Input: part model. Units: mm. Frame: model coordinates. Face numbers are marked on the shaded views. A direction names the side the tool comes from. Give positions to 0.01 mm unless a question says otherwise; leave off trailing zeros. Loops run counter-clockwise (first coordinate to the right, second up) from the corner with the lowest first, then second, coordinate; pieces in that order, holes last. Notation, with made-up numbers: (44, 10.25) -> (78, 10.25) arc R25 ccw to (78, 48.25) -> close; hole circle Ø11 at (4, 49). An arc over 180 degrees is marked (long way). One line per question, with ' | ' between items.
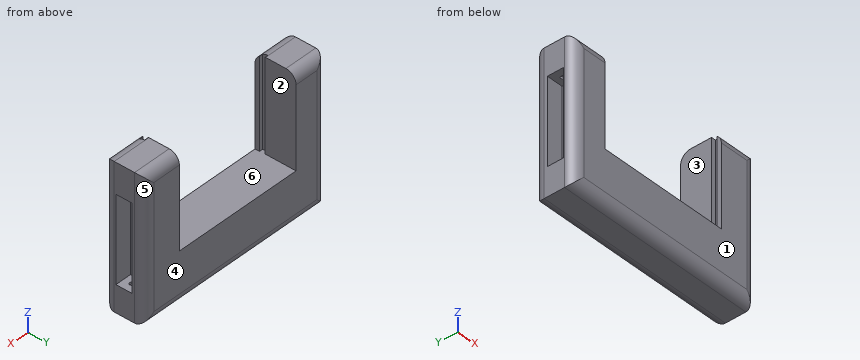
from build123d import *

# Parameters (mm, degrees)
SKETCH1_W           = 50
SKETCH1_H           = 35
BOSS_EXTRUDE1_DEPTH = 10
SKETCH2_W           = 34
SKETCH2_H           = 1.3
CUT_EXTRUDE1_DEPTH  = 22.5
SKETCH3_W           = 15
SKETCH3_H           = 7.598280995
CUT_EXTRUDE2_DEPTH  = 22.5
SKETCH4_W           = 17.2
SKETCH4_H           = 7.598280995
CUT_EXTRUDE3_DEPTH  = 22.5
SKETCH5_W           = 13.5
SKETCH5_H           = 1.101719005
CUT_EXTRUDE4_DEPTH  = 22.5
SKETCH6_W           = 18.6
SKETCH6_H           = 1.101719005
CUT_EXTRUDE5_DEPTH  = 22.5
SKETCH7_W           = 21
SKETCH7_H           = 4
CUT_EXTRUDE6_DEPTH  = 4
SKETCH8_R           = 0.5
CUT_EXTRUDE7_DEPTH  = 0.5
SKETCH9_R           = 0.5
CUT_EXTRUDE8_DEPTH  = 0.5
SKETCH10_W          = 21
SKETCH10_H          = 4
CUT_EXTRUDE9_DEPTH  = 4
SKETCH11_R          = 0.5
CUT_EXTRUDE10_DEPTH = 0.5
SKETCH12_R          = 0.5
CUT_EXTRUDE11_DEPTH = 0.5
FILLET1_R           = 2.5


with BuildPart() as part:
    # Sketch1 → Boss-Extrude1 (new body)
    with BuildSketch(Plane(origin=(0, 0, 0), x_dir=(1, 0, 0), z_dir=(0, 1, 0))):
        with Locations((-1.379996057, -3.323754789)):
            Rectangle(SKETCH1_W, SKETCH1_H)
    extrude(amount=BOSS_EXTRUDE1_DEPTH)

    # Sketch2 → Cut-Extrude1 (cut)
    with BuildSketch(Plane.XY.offset(20.823754789)):
        with Locations((-1.867795916, 1.751719005)):
            Rectangle(SKETCH2_W, SKETCH2_H)
    extrude(amount=-CUT_EXTRUDE1_DEPTH, mode=Mode.SUBTRACT)

    # Sketch3 → Cut-Extrude2 (cut)
    with BuildSketch(Plane.XY.offset(20.823754789)):
        with Locations((6.564825068, 6.200859503)):
            Rectangle(SKETCH3_W, SKETCH3_H)
    extrude(amount=-CUT_EXTRUDE2_DEPTH, mode=Mode.SUBTRACT)

    # Sketch4 → Cut-Extrude3 (cut)
    with BuildSketch(Plane.XY.offset(20.823754789)):
        with Locations((-9.535174932, 6.200859503)):
            Rectangle(SKETCH4_W, SKETCH4_H)
    extrude(amount=-CUT_EXTRUDE3_DEPTH, mode=Mode.SUBTRACT)

    # Sketch5 → Cut-Extrude4 (cut)
    with BuildSketch(Plane.XY.offset(20.823754789)):
        with Locations((7.329591682, 0.550859503)):
            Rectangle(SKETCH5_W, SKETCH5_H)
    extrude(amount=-CUT_EXTRUDE4_DEPTH, mode=Mode.SUBTRACT)

    # Sketch6 → Cut-Extrude5 (cut)
    with BuildSketch(Plane.XY.offset(20.823754789)):
        with Locations((-8.720408318, 0.550859503)):
            Rectangle(SKETCH6_W, SKETCH6_H)
    extrude(amount=-CUT_EXTRUDE5_DEPTH, mode=Mode.SUBTRACT)

    # Sketch7 → Cut-Extrude6 (cut)
    with BuildSketch(Plane.ZY.offset(26.379996057)):
        with Locations((3.348440288, 4.718765764)):
            Rectangle(SKETCH7_W, SKETCH7_H)
    extrude(amount=-CUT_EXTRUDE6_DEPTH, mode=Mode.SUBTRACT)

    # Sketch8 → Cut-Extrude7 (cut)
    with BuildSketch(Plane.XY.offset(-7.151559712)):
        with Locations((-24.165741094, 4.777186657)):
            Circle(SKETCH8_R)
    extrude(amount=-CUT_EXTRUDE7_DEPTH, mode=Mode.SUBTRACT)

    # Sketch9 → Cut-Extrude8 (cut)
    with BuildSketch(Plane(origin=(0, 0, 13.848440288), x_dir=(-1, 0, 0), z_dir=(0, 0, -1))):
        with Locations((24.247358315, 4.819765538)):
            Circle(SKETCH9_R)
    extrude(amount=-CUT_EXTRUDE8_DEPTH, mode=Mode.SUBTRACT)

    # Sketch10 → Cut-Extrude9 (cut)
    with BuildSketch(Plane(origin=(23.620003943, 0, 0), x_dir=(0, 0, -1), z_dir=(1, 0, 0))):
        with Locations((-2.904513536, 4.904491876)):
            Rectangle(SKETCH10_W, SKETCH10_H)
    extrude(amount=-CUT_EXTRUDE9_DEPTH, mode=Mode.SUBTRACT)

    # Sketch11 → Cut-Extrude10 (cut)
    with BuildSketch(Plane(origin=(0, 0, 13.404513536), x_dir=(-1, 0, 0), z_dir=(0, 0, -1))):
        with Locations((-21.490093602, 4.986179228)):
            Circle(SKETCH11_R)
    extrude(amount=-CUT_EXTRUDE10_DEPTH, mode=Mode.SUBTRACT)

    # Sketch12 → Cut-Extrude11 (cut)
    with BuildSketch(Plane.XY.offset(-7.595486464)):
        with Locations((21.482332732, 4.892682942)):
            Circle(SKETCH12_R)
    extrude(amount=-CUT_EXTRUDE11_DEPTH, mode=Mode.SUBTRACT)

    # Fillet1
    fillet1_edges = [part.edges().sort_by_distance(p)[0] for p in [
        (-22.200202188, 0, 20.823754789),
        (18.849797812, 0, 20.823754789),
        (-26.379996057, 0, 3.323754789),
        (-26.379996057, 10, 3.323754789),
        (-22.257585495, 10, 20.823754789),
        (18.842414505, 10, 20.823754789),
        (-1.379996057, 0, -14.176245211),
        (-1.379996057, 10, -14.176245211),
        (23.620003943, 0, 3.323754789),
        (23.620003943, 10, 3.323754789),
    ]]
    fillet(fillet1_edges, radius=FILLET1_R)


solid = part.part
1. Section query C-C (x = 16.5). Output: boundary loops of the cut face in (y, z), then the cut area to 3 significant figures.
Determined:
outline: (0, -11.68) arc R2.5 ccw to (2.5, -14.18) -> (7.5, -14.18) arc R2.5 ccw to (10, -11.68) -> (10, 18.32) arc R2.5 ccw to (7.5, 20.82) -> (2.5, 20.82) arc R2.5 ccw to (0, 18.32) -> close | area: 345 mm2
2. Pin query (flat end, axial travel): P1, Ø3, axis at y = 2, z = -9.5, coming from the +X side; P2, Ø0.9, axis at y = 0.5, z = 14.5, coming from the +X side; P3, Ø1, axis at x = -0.5, y = 6, coming from the +Z side; P4, Ø2, axis at x = -11.5, y = 9, coming from the -Z side. Return the tip coordinate at first contact, or that it passes through.
Determined:
P1: stops at x = 23.62 | P2: stops at x = 23.08 | P3: stops at z = -1.68 | P4: stops at z = -14.13
3. Section query A-A (z = 4). Output: boundary loops of the cut face in (x, y).
Determined:
outline: (-26.38, 2.5) arc R2.5 ccw to (-23.88, 0) -> (-18.02, 0) -> (-18.02, 1.1) -> (-18.87, 1.1) -> (-18.87, 2.4) -> (-18.14, 2.4) -> (-18.14, 10) -> (-23.88, 10) arc R2.5 ccw to (-26.38, 7.5) -> (-26.38, 6.72) -> (-22.38, 6.72) -> (-22.38, 2.72) -> (-26.38, 2.72) -> close; (14.06, 2.4) -> (15.13, 2.4) -> (15.13, 1.1) -> (14.08, 1.1) -> (14.08, 0) -> (21.12, 0) arc R2.5 ccw to (23.62, 2.5) -> (23.62, 2.9) -> (19.62, 2.9) -> (19.62, 6.9) -> (23.62, 6.9) -> (23.62, 7.5) arc R2.5 ccw to (21.12, 10) -> (14.06, 10) -> close
4. Reachability of the marked faces 1, 2 and 3 from +Z, -Z, +X, -X, +Y, -Y: full face, straight path, thin tool, end or side. Return the list, or none.
Determined:
face 1: +Z, -Z, +X, -X, -Y | face 2: +Z, +Y | face 3: +Z, +Y, -Y
5. Pull-direction query (X, two-part tool) for the marked faces 4, 5 and 6; classes: pulls with the +X half, pulls with the -X half, needs draft (parallel to the pull), parting line crosses it, or undercut.
Determined:
face 4: needs draft | face 5: pulls with the +X half | face 6: undercut
6. Section query D-D (x = -13). Output: boundary loops of the cut face in (y, z), then the cut area to 3 significant figures.
Determined:
outline: (0, -11.68) arc R2.5 ccw to (2.5, -14.18) -> (7.5, -14.18) arc R2.5 ccw to (10, -11.68) -> (10, -1.68) -> (0, -1.68) -> close | area: 122 mm2
7. Ray query, line 1 along Z through (x, y) = (-22.5, 5.25); line 2 along X through (y, z) = (7.25, 1.5); line 3 along Z through (x, y) = (11, 5.5). Return the intervals inside material, ascending. Write a range as from..to.
Determined:
line 1: z = -14.18..-7.15, 13.85..20.82 | line 2: x = -26.38..-18.14, 14.06..23.62 | line 3: z = -14.18..-1.68
8. Section query B-B (y = 3.5). Output: boundary loops of the cut face in (x, z).
Determined:
outline: (-26.38, -14.18) -> (23.62, -14.18) -> (23.62, -7.6) -> (19.62, -7.6) -> (19.62, 13.4) -> (23.62, 13.4) -> (23.62, 20.82) -> (14.06, 20.82) -> (14.06, -1.68) -> (-18.14, -1.68) -> (-18.14, 20.82) -> (-26.38, 20.82) -> (-26.38, 13.85) -> (-22.38, 13.85) -> (-22.38, -7.15) -> (-26.38, -7.15) -> close
